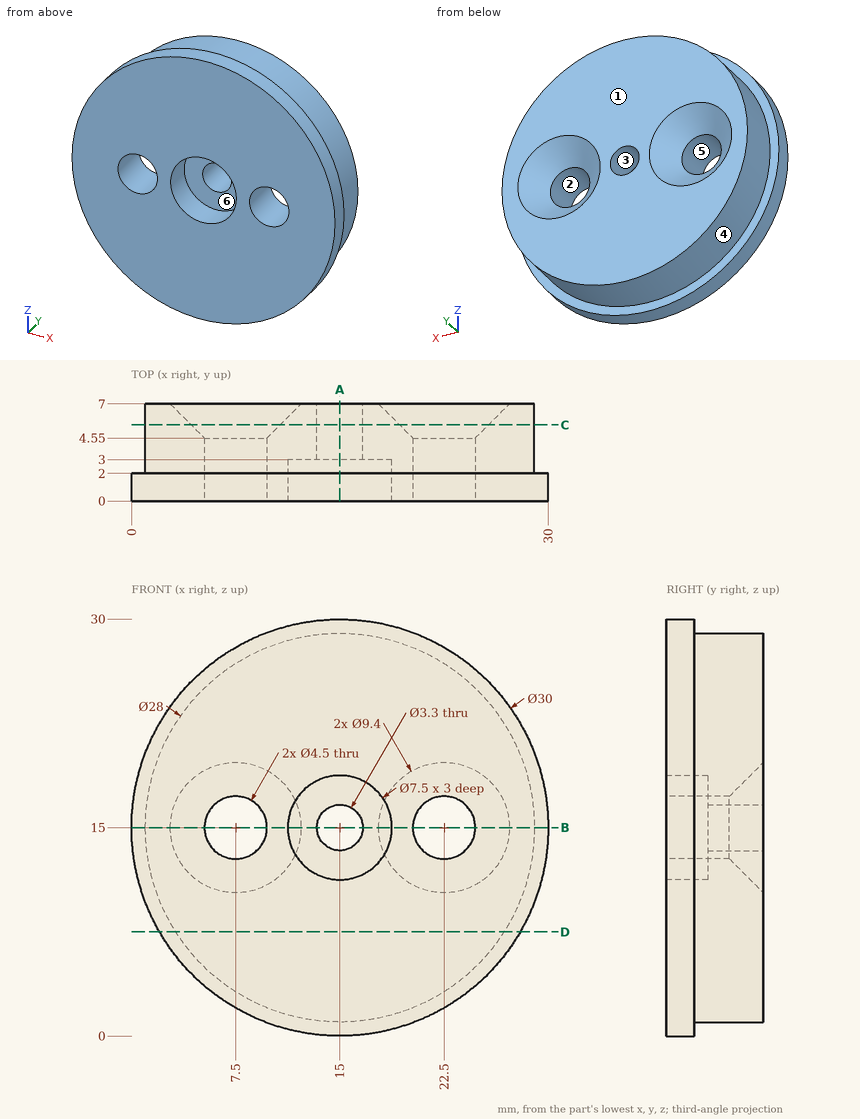
Design review of the part shown in the three views and the two pictorial views. Dimensions are in mm from the part's minimum x, y and z. A direction names the side the tool comes from. Give positions to 0.01 mm unless a question says otherwise; leave off trailing zeros. Write each loop counter-clockwise with the first axis right and the second up, starting at its lowest first coordinate (ties: lowest second). Pieces come first, ordered by that corner, then holes.
Item 1: Machinability: for the marked faces 5 and 6, which of the approach directions +Z, -Z, +X, -X, +Y, -Y give a long, thin tool a straight path to every point of the face, cutting with its end or side? Answer none if there is none.
Item 2: Take a section at B-B (z = 15). Give the boundary of the cut face in (x, y), and give its area (3 significant figures).
Item 3: The part is to be moulded in two halves that separate along Z. For the marked faces 1, 2, 3 and 4, say which applies: +Z half, -Z half, draft (parallel to the pull), parting line (faces both ways), or undercut.
Item 4: Take a section at C-C (y = 5.5). Give the boundary of the cut face in (x, z), and give its area (3 significant figures).
Item 5: Take a section at D-D (z = 7.5). Give the boundary of the cut face in (x, y), and give its area (3 significant figures).
Item 6: Wall thickness on probe 1 along X at (y, z) = (3.5, 14.25); probe 2 along Z at (x, y) = (15, 5.55); probe 3 along Z at (x, y) = (15, 1.55): over which ranges is each line inside the solid? List them lowest first.
Item 7: Take a section at A-A (x = 15). Give the boundary of the cut face in (y, z).
Item 8: Insertion check: P1, Ø2.5, axis at x = 22.5, z = 15, coming from the +Y side; P2, Ø1, axis at y = 6, z = 25.5, coming from the +X side; P3, Ø2, axis at y = 6, z = 15, coming from the +X side; P4, Ø1.5, axis at x = 7.5, y = 4, coming from the +Z side. Each pin has a flat end and moves straight along its axis. Give the tip position at first contact, or say it passes through.
Established:
1. face 5: +Y, -Y
1. face 6: -Y
2. outline: (0, 0) - (5.25, 0) - (5.25, 4.55) - (2.8, 7) - (1, 7) - (1, 2) - (0, 2) - close; (9.75, 0) - (11.25, 0) - (11.25, 3) - (13.35, 3) - (13.35, 7) - (12.2, 7) - (9.75, 4.55) - close; (16.65, 3) - (18.75, 3) - (18.75, 0) - (20.25, 0) - (20.25, 4.55) - (17.8, 7) - (16.65, 7) - close; (24.75, 0) - (30, 0) - (30, 2) - (29, 2) - (29, 7) - (27.2, 7) - (24.75, 4.55) - close
2. area: 89.3 mm2
3. face 1: draft
3. face 2: undercut
3. face 3: undercut
3. face 4: parting line
4. outline: circle Ø28 at (15, 15); hole circle Ø6.4 at (7.5, 15); hole circle Ø3.3 at (15, 15); hole circle Ø6.4 at (22.5, 15)
4. area: 543 mm2
5. outline: (2.01, 0) - (27.99, 0) - (27.99, 2) - (26.82, 2) - (26.82, 7) - (3.18, 7) - (3.18, 2) - (2.01, 2) - close
5. area: 170 mm2
6. probe 1: x = 1.02 to 5.38, 9.62 to 13.53, 16.47 to 20.38, 24.62 to 28.98
6. probe 2: z = 1 to 13.35, 16.65 to 29
6. probe 3: z = 0 to 11.25, 18.75 to 30
7. outline: (0, 0) - (2, 0) - (2, 1) - (7, 1) - (7, 13.35) - (3, 13.35) - (3, 11.25) - (0, 11.25) - close; (0, 18.75) - (3, 18.75) - (3, 16.65) - (7, 16.65) - (7, 29) - (2, 29) - (2, 30) - (0, 30) - close
8. P1: passes through
8. P2: stops at x = 24.8
8. P3: stops at x = 29
8. P4: stops at z = 27.27
